Here's how the part is built. I have some questions about the finished solid (model axes, mm). A direction names the side the tool comes from. Round coordinates to 2 decimals unless told otherwise and drop trailing zeros. Write each loop counter-clockwise with the first axis right and the second up, starting at its lowest first coordinate (ties: lowest second). Pieces come first, ordered by that corner, then holes. Notation, with made-up numbers: M 17,-12 L 35,-12 A12 ccw 35,-4 Z; hole C 62,5.25 d4. An arc over 180 degrees is marked long. Write item = value, one per line. Start each with the question number.
(1) If we mould it in two halves opening along Y, with no side actions, what happens to faces 1 (the cylindrical face through (-11, -14, -20.6)), 2 (the flat face through (-2.91, 0.99, 5.34)), 3 (the flat face through (-1, 0, -6)), 4 (the flat face through (-11, -8, -19.1))? For each: released by +Y, released by -Y, zero draft, split by the parting line, or undercut.
(2) I want a section at D-D (x = 8.75). List the corners of the cut face in (y, z) for me, and give its area (3 significant figures).
(3) On a 3-axis mill with a long thin cutter (end or side, diameter ignored), from which of +Z, -Z, +X, -X, +Y, -Y can I reach the whole of each face in a straight line? I mean faces 5 (the flat face through (-10, -13.8, -19.5)), 6 (the cylindrical face through (7.057, 0.986, 10.894)), 7 (the flat face through (0, 1, -21)), 8 (the flat face through (-11, -8, -22.1)). Say none if no direction works.
(4) I want a section at C-C (z = -18.5). List the corners of the cut face in (x, y) for me, and give its area (3 significant figures).
(5) I want a section at A-A (y = -23). List the corners of the cut face in (x, z) for me.
(6) Will these pins go through, and if not, where does the flat tip stop? pin 1 Ø4 at (x, y) = (-9.5, -3.5) entering from +Z; pin 2 Ø4 at (y, z) = (-9, -17.5) entering from +X; pin 3 Ø5 at (x, z) = (-3, -10) entering from -Y.
(7) I want a section at B-B (x = -0.75). List the corners of the cut face in (y, z) for me.
(8) I need wall thicknesses on line 1 along Z through (x, y) = (-11.25, -23); line 2 along Y through (x, z) = (-1, -24); line 3 along X through (y, z) = (-7.5, -18). Which ranges of each line are inside material? Lowest first, please.
```python
from build123d import *

# Parameters (mm, degrees)
SKETCH1_R              = 1.5
BOSS_EXTRUDE1_DEPTH    = 2
SKETCH2_W              = 2
SKETCH2_H              = 21.859501482
BOSS_EXTRUDE3_DEPTH    = 30
CUT_EXTRUDE1_START     = -12
CUT_EXTRUDE1_OUTLINE_R = 1.5
CUT_EXTRUDE1_DEPTH     = 2
CUT_EXTRUDE2_DEPTH     = 30


# Read off the part's stored shape, not the designer's step: Cut-Extrude1
with BuildPart() as part:
    # Sketch1 → Boss-Extrude1 (new body)
    with BuildSketch(Plane(origin=(0, 0, 0), x_dir=(1, 0, 0), z_dir=(0, 1, 0))):
        Polygon((-10, 30.6), (0, 30.6), (0, 11.116380148), (12.920279645, -14.539262377), (3.988919615, -19.037129429), (-10, 8.740498518), align=None)
        with Locations(Location((0, 0, 0), (0, 0, 270))):
            Circle(SKETCH1_R, mode=Mode.SUBTRACT)
        with Locations(Location((6.043245871, -12, 0), (0, 0, 270))):
            Circle(SKETCH1_R, mode=Mode.SUBTRACT)
    extrude(amount=BOSS_EXTRUDE1_DEPTH)

    # Sketch2 → Boss-Extrude3 (add)
    with BuildSketch(Plane(origin=(0, 2, 0), x_dir=(1, 0, 0), z_dir=(0, 1, 0))):
        with Locations((-11, 19.670249259)):
            Rectangle(SKETCH2_W, SKETCH2_H)
    extrude(amount=-BOSS_EXTRUDE3_DEPTH)

    # Cut-Extrude1 outline → Cut-Extrude1 (cut)
    with BuildSketch(Plane.YZ.offset(CUT_EXTRUDE1_START)):
        with Locations((-23, -20.6)):
            Circle(CUT_EXTRUDE1_OUTLINE_R)
    extrude(amount=CUT_EXTRUDE1_DEPTH, mode=Mode.SUBTRACT)

    # Sketch4 → Cut-Extrude2 (cut)
    with BuildSketch(Plane.ZY.offset(12)):
        with BuildLine():
            Line((-19.1, -3.5), (-19.1, -12.5))
            ThreePointArc((-19.1, -12.5), (-20.6, -14), (-22.1, -12.5))
            Line((-22.1, -12.5), (-22.1, -3.5))
            ThreePointArc((-22.1, -3.5), (-20.6, -2), (-19.1, -3.5))
        make_face()
    extrude(amount=-CUT_EXTRUDE2_DEPTH, mode=Mode.SUBTRACT)


solid = part.part
```
Returned:
q1.face_1 = undercut
q1.face_2 = zero draft
q1.face_3 = released by -Y
q1.face_4 = undercut
q2.outline = M 0,6.26 L 2,6.26 L 2,16.64 L 0,16.64 Z
q2.area = 20.8 mm²
q3.face_5 = +Z, -Z, +X, -Y
q3.face_6 = +Y, -Y
q3.face_7 = -Z, +X, +Y, -Y
q3.face_8 = +X, -X
q4.outline = M -12,-28 L -10,-28 L -10,0 L 0,0 L 0,2 L -12,2 Z
q4.area = 80.0 mm²
q5.outline = M -12,-30.6 L -10,-30.6 L -10,-22.1 L -12,-22.1 Z; M -12,-19.1 L -10,-19.1 L -10,-8.74 L -12,-8.74 Z
q6.pin_1 = -8.74
q6.pin_2 = -10
q6.pin_3 = 0
q7.outline = M 0,-30.6 L 2,-30.6 L 2,-1.3 L 0,-1.3 Z; M 0,1.3 L 2,1.3 L 2,9.63 L 0,9.63 Z
q8.line_1 = -30.6 to -22.1, -19.1 to -8.74
q8.line_2 = 0 to 2
q8.line_3 = -12 to -10
